```python
from build123d import *

# Parameters (mm, degrees)
SKETCH2_W                      = 89
SKETCH2_H                      = 72
BOSS_EXTRUDE1_DEPTH            = 6
CBORE_FOR_M4_SHCS1_D           = 4.3
CBORE_FOR_M4_SHCS1_CBORE_D     = 8
CBORE_FOR_M4_SHCS1_CBORE_DEPTH = 4
M5_CLEARANCE_HOLE1_D           = 5.3
FILLET1_R                      = 3


with BuildPart() as part:
    # Sketch2 → Boss-Extrude1 (new body)
    with BuildSketch(Plane(origin=(0, 0, 0), x_dir=(1, 0, 0), z_dir=(0, 1, 0))):
        Rectangle(SKETCH2_W, SKETCH2_H)
    extrude(amount=BOSS_EXTRUDE1_DEPTH)

    # CBORE for M4 SHCS1 (through all)
    with Locations(Plane(origin=(0, 0, 0), x_dir=(-1, 0, 0), z_dir=(0, -1, 0))):
        with Locations((-16, -16), (-16, 16), (16, 16), (16, -16)):
            CounterBoreHole(CBORE_FOR_M4_SHCS1_D / 2, CBORE_FOR_M4_SHCS1_CBORE_D / 2, CBORE_FOR_M4_SHCS1_CBORE_DEPTH)

    # M5 Clearance Hole1 (through all)
    with Locations(Plane(origin=(0, 6, 0), x_dir=(1, 0, 0), z_dir=(0, 1, 0))):
        with Locations((-40, 6.34428877), (40, 6.34428877)):
            Hole(M5_CLEARANCE_HOLE1_D / 2)

    # Fillet1
    fillet1_edges = [part.edges().sort_by_distance(p)[0] for p in [
        (-44.5, 3, -36),
        (44.5, 3, -36),
        (44.5, 3, 36),
        (-44.5, 3, 36),
    ]]
    fillet(fillet1_edges, radius=FILLET1_R)


solid = part.part
```
Geometry check sheet. Reference: the model listing, model coordinates, mm. A direction names the side the tool comes from. Round coordinates to 2 decimals unless told otherwise and drop trailing zeros. Order: outer loops, then holes, each group sorted by start corner. A loop starts at its lowest first (then second) coordinate and runs counter-clockwise, first axis right, second up. Notation, with made-up numbers: M -33.75,-13.75 L -20.75,-13.75 A16 cw -20.75,-7.75 Z; hole C 50,78 d7. An arc over 180 degrees is marked long. Answer as CSV lines item,"result".
1) Tool access check on faces 1 (the face through (18.95, 1.97, -18.7)), 2 (the face through (-15.01, 5.01, -14.09)). Record the directions out of +Z, -Z, +X, -X, +Y, -Y that give a thin tool (end or side, any length) a straight path to the whole face; none if there is none.
Entries:
face 1,"-Y"
face 2,"+Y, -Y"
2) Sectioned sample at A-A on x = -16. Record the cut outline in (y, z).
Entries:
outline,"M 0,-36 L 6,-36 L 6,-18.15 L 4,-18.15 L 4,-20 L 0,-20 Z; M 0,-12 L 4,-12 L 4,-13.85 L 6,-13.85 L 6,13.85 L 4,13.85 L 4,12 L 0,12 Z; M 0,20 L 4,20 L 4,18.15 L 6,18.15 L 6,36 L 0,36 Z"
3) Mould release check, pull along X, two halves, no side actions. Record for faces 3 (the face through (-43.64, 3.04, -35.1)), 4 (the face through (-1, 0, -1)), 5 (the face through (-12, 2, 16)), 6 (the face through (14, 4, -14)): +X half, -X half, draft (parallel to the pull), parting line (faces both ways), or undercut.
Entries:
face 3,"-X half"
face 4,"draft"
face 5,"undercut"
face 6,"undercut"
4) Sectioned sample at C-C on x = 40. Record the cut outline in (y, z), and give its area (3 significant figures).
Entries:
outline,"M 0,-36 L 6,-36 L 6,-8.99 L 0,-8.99 Z; M 0,-3.69 L 6,-3.69 L 6,36 L 0,36 Z"
area,"400 mm2"
5) Thickness scan on probe 1 along X at (y, z) = (1.15, 16); probe 2 along Z at (x, y) = (-16, 1); probe 3 along X at (y, z) = (4.5, 16). Record the ranges inside material, lowest first. Write a range as [from, to].
Entries:
probe 1,"[-44.5, -20], [-12, 12], [20, 44.5]"
probe 2,"[-36, -20], [-12, 12], [20, 36]"
probe 3,"[-44.5, -18.15], [-13.85, 13.85], [18.15, 44.5]"
6) Sectioned sample at B-B on z = -16. Record the cut outline in (x, y).
Entries:
outline,"M -44.5,0 L -20,0 L -20,4 L -18.15,4 L -18.15,6 L -44.5,6 Z; M -13.85,4 L -12,4 L -12,0 L 12,0 L 12,4 L 13.85,4 L 13.85,6 L -13.85,6 Z; M 18.15,4 L 20,4 L 20,0 L 44.5,0 L 44.5,6 L 18.15,6 Z"
7) Gauge pin test, flat ends, axial feed: pin 1 Ø10.5 at (x, z) = (16, -16) entering from -Y; pin 2 Ø7 at (x, z) = (16, 16) entering from -Y; pin 3 Ø2.5 at (x, z) = (-16, 16) entering from -Y. Record the tip position at first contact, or that the pin passes through.
Entries:
pin 1,"y = 0"
pin 2,"y = 4"
pin 3,"through"
8) Sectioned sample at D-D on y = 2.3. Record the cut outline in (x, z), and give its area (3 significant figures).
Entries:
outline,"M -44.5,-33 A3 ccw -41.5,-36 L 41.5,-36 A3 ccw 44.5,-33 L 44.5,33 A3 ccw 41.5,36 L -41.5,36 A3 ccw -44.5,33 Z; hole C -40,-6.34 d5.3; hole C -16,-16 d8; hole C -16,16 d8; hole C 16,-16 d8; hole C 16,16 d8; hole C 40,-6.34 d5.3"
area,"6,160 mm2"
